Geometry: see drawing. Coordinates: mm, zero at the bounding-box minimum. A direction names the side the tool comes from. Round coordinates to 2 decimals unless told otherwise and drop trailing zeros. Order: outer loops, then holes, each group sorted by start corner. A loop starts at its lowest first (then second) coordinate and runs counter-clockwise, first axis right, second up. Notation, with made-up numbers: (34.5, 13) -> (45.5, 13) arc R17 cw to (45.5, 32) -> close; hole circle Ø10 at (83, -2.75). An arc over 180 degrees is marked (long way). Put each result on its own line as item: value.
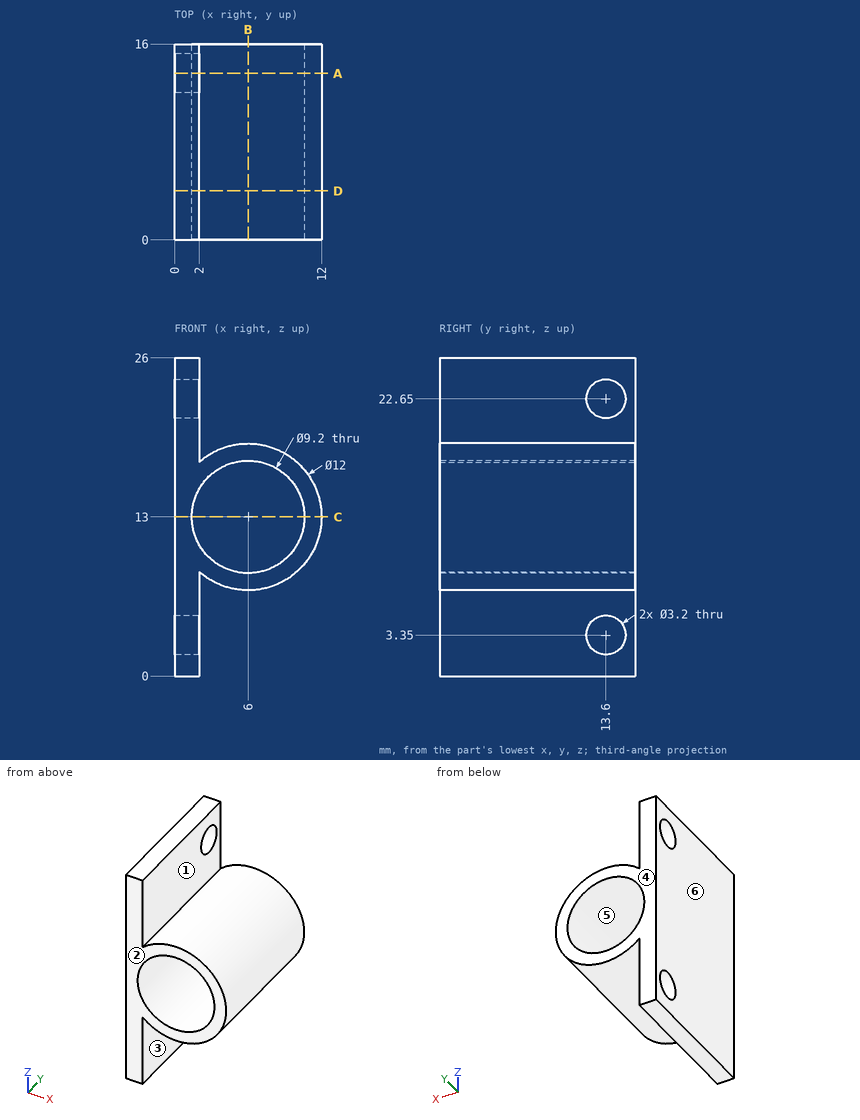
1. Set-up query: the marked faces 1, 2 and 3. Return all of +Z, -Z, +X, -X, +Y, -Y with unobstructed straight access to the full face (end or side cutting, diameter ignored); none if empty.
Ans:
face 1: +Z, +Y, -Y
face 2: +Z, -Z, +X, -X, -Y
face 3: -Z, +Y, -Y
2. Draft query along X for the marked faces 4, 5 and 6. Return one class per face: +X half, -X half, draft (parallel to the pull), parting line (faces both ways), or undercut.
Ans:
face 4: draft
face 5: undercut
face 6: -X half
3. Cut plane C-C on z = 13. Return loops of the section in (x, y).
Ans:
outline: (0, 0) -> (1.4, 0) -> (1.4, 16) -> (0, 16) -> close; (10.6, 0) -> (12, 0) -> (12, 16) -> (10.6, 16) -> close
4. Cut plane A-A on y = 13.6. Return loops of the section in (x, z).
Ans:
outline: (0, 0) -> (2, 0) -> (2, 1.75) -> (0, 1.75) -> close; (0, 4.95) -> (2, 4.95) -> (2, 8.53) arc R6 ccw (long way) to (2, 17.47) -> (2, 21.05) -> (0, 21.05) -> close; (0, 24.25) -> (2, 24.25) -> (2, 26) -> (0, 26) -> close; hole circle Ø9.2 at (6, 13)
5. Contact query for flat-ended pins moving along their axis: P1, Ø1, axis at x = 3, y = 13.5, coming from the -Z side; P2, Ø2.5, axis at y = 10, z = 5.5, coming from the +X side; P3, Ø1, axis at x = 8.5, y = 11, coming from the +Z side. Output: stop coordinate, or through.
Ans:
P1: z = 7.55
P2: x = 2
P3: z = 18.66
6. Material intervals for probe 1 along Y at (x, z) = (1.05, 3.35); probe 2 along Z at (x, y) = (6, 13); probe 3 along X at (y, z) = (6, 8), sorted ascending.
Ans:
probe 1: 0 to 12, 15.2 to 16
probe 2: 7 to 8.4, 17.6 to 19
probe 3: 0 to 2, 2.68 to 9.32
7. Cut plane B-B on x = 6. Return loops of the section in (y, z).
Ans:
outline: (0, 7) -> (16, 7) -> (16, 8.4) -> (0, 8.4) -> close; (0, 17.6) -> (16, 17.6) -> (16, 19) -> (0, 19) -> close
8. Cut plane D-D on y = 4. Return loops of the section in (x, z), and give its area (3 significant figures).
Ans:
outline: (0, 0) -> (2, 0) -> (2, 8.53) arc R6 ccw (long way) to (2, 17.47) -> (2, 26) -> (0, 26) -> close; hole circle Ø9.2 at (6, 13)
area: 86.2 mm²
